Geometry: see drawing. Coordinates: mm, zero at the bounding-box minimum. Give positions to 0.01 mm unless a question says otherwise; leave off trailing zeros. Write each loop counter-clockwise with the first axis right and the second up, starting at its lowest first coordinate (ties: lowest second). Pieces come first, ordered by that corner, then holes. Notation, with made-up numbers: M 66,73.5 L 95,73.5 A27 cw 95,103.5 Z; hole C 65.25,-20 d3. An arc over 180 degrees is marked long. Use a Markdown table: item, result. Add a question column.
1) Section D-D on y = 2.75. Return the cut outline in (x, z).
2) Section C-C on y = 17.5. Return the cut outline in (x, z).
3) Section B-B on z = 2.35. Return the cut outline in (x, y).
4) Section A-A on x = 0.25. Return the cut outline in (y, z).
5) Line query: line 1 (Z direction, x = 0.4, y = 15); line 2 (Z direction, x = 0.45, y = 7.5) (1 decimal); line 3 (Y direction, x = 0.15, z = 0.2) (1 decimal). Output: solid intervals per line, ascending.
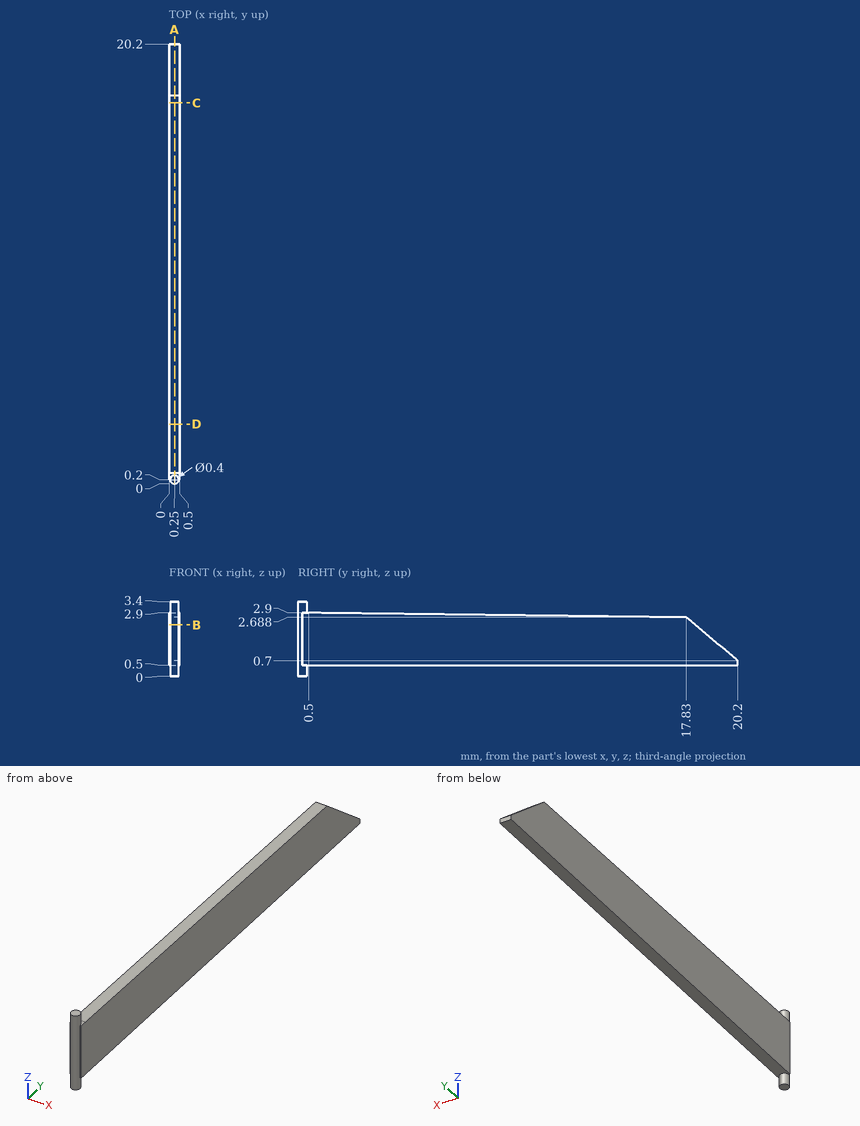
Found:
| question | item | result |
|---|---|---|
| 1 | outline | M 0,0.5 L 0.5,0.5 L 0.5,2.87 L 0,2.87 Z |
| 2 | outline | M 0,0.5 L 0.5,0.5 L 0.5,2.69 L 0,2.69 Z |
| 3 | outline | M 0,0.2 L 0.05,0.2 A0.2 ccw 0.45,0.2 L 0.5,0.2 L 0.5,18.23 L 0,18.23 Z |
| 4 | outline | M 0,0 L 0.4,0 L 0.4,0.5 L 20.2,0.5 L 20.2,0.7 L 17.83,2.69 L 0.5,2.9 L 0.4,2.9 L 0.4,3.4 L 0,3.4 Z |
| 5 | line 1 | 0.5 to 2.72 |
| 5 | line 2 | 0.5 to 2.8 |
| 5 | line 3 | 0 to 0.4 |
